Here's how the part is built. I have some questions about the finished solid (model axes, mm). Face numbers are marked on the shaded views. A direction names the side the tool comes from. Round coordinates to 2 decimals unless told otherwise and drop trailing zeros. Order: outer loops, then holes, each group sorted by start corner. A loop starts at its lowest first (then second) coordinate and runs counter-clockwise, first axis right, second up. Notation, with made-up numbers: (77, 22) -> (121, 22) arc R27 ccw to (121, 41) -> close; hole circle Ø1 at (71.25, -18). An arc over 180 degrees is marked (long way). Answer in a Markdown table with one row per item.
Solid Edge part; units mm, degrees
sketch "Sketch1" plane through (0, 0, 0) normal (0, 0, 1) x (1, 0, 0)
  line L0 (-22.86, 0) -> (22.86, 0)
  line L1 (22.86, 0) -> (22.86, 21.336)
  line L2 (22.86, 21.336) -> (-22.86, 21.336)
  line L3 (-22.86, 21.336) -> (-22.86, 0)
extrude "Protrusion1" add sketch "Sketch1" along normal blind 3.81
sketch "Sketch2" plane through (0, 10.668, 3.81) normal (0, 0, 1) x (1, 0, 0)
  circle A0 centre (12.7, 0) radius 8.001
  circle A1 centre (-12.7, 0) radius 8.001
  dimension "D1" = 12.7
  dimension "D2" = 12.7
extrude "ExtrudedProtrusion_2" add sketch "Sketch2" along normal blind 11.938
hole "Hole_1" at (20.32, 18.796, 3.81) direction (0, 0, -1) diameter 3.175 end up to next
hole "Hole1" at (-20.32, 2.54, 3.81) direction (0, 0, -1) diameter 3.175 end up to next
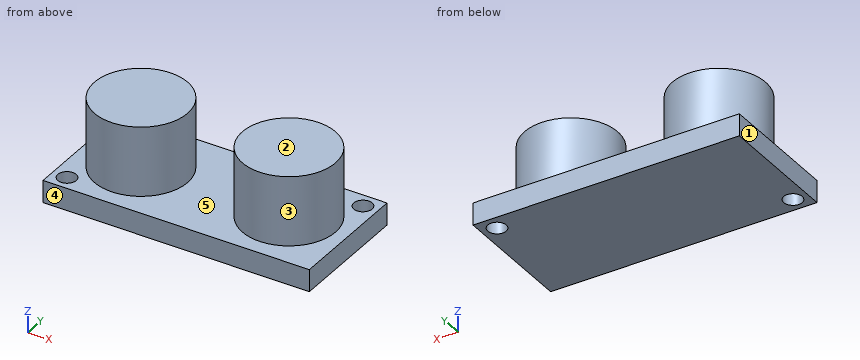
1. Suppose I cut it at A-A on y = 15.5. Write out the boundary of the cut face in (x, z), then the cut area to 3 significant figures.
Numbers:
| item | result |
|---|---|
| outline | (-22.86, 0) -> (22.86, 0) -> (22.86, 3.81) -> (19.08, 3.81) -> (19.08, 15.75) -> (6.32, 15.75) -> (6.32, 3.81) -> (-6.32, 3.81) -> (-6.32, 15.75) -> (-19.08, 15.75) -> (-19.08, 3.81) -> (-22.86, 3.81) -> close |
| area | 479 mm2 |
2. Suppose I cut it at C-C on z = 7. Write out the boundary of the cut face in (x, y).
Numbers:
| item | result |
|---|---|
| outline | circle Ø16 at (-12.7, 10.67); circle Ø16 at (12.7, 10.67) |
3. Suppose I cut it at D-D on x = 10. Write out the boundary of the cut face in (y, z), then the cut area to 3 significant figures.
Numbers:
| item | result |
|---|---|
| outline | (0, 0) -> (21.34, 0) -> (21.34, 3.81) -> (18.2, 3.81) -> (18.2, 15.75) -> (3.14, 15.75) -> (3.14, 3.81) -> (0, 3.81) -> close |
| area | 261 mm2 |
4. Please list where these lines run through material, in increasing order: line 1 along Y through (x, z) = (-20.32, 2.2); line 2 along Y through (x, z) = (20.32, 2.45); line 3 along X through (y, z) = (2.54, 1.2).
Numbers:
| item | result |
|---|---|
| line 1 | y = 0 to 0.95, 4.13 to 21.34 |
| line 2 | y = 0 to 17.21, 20.38 to 21.34 |
| line 3 | x = -22.86 to -21.91, -18.73 to 22.86 |
5. We'd pull the mould along X, two halves only. Please class the marked faces 1, 2 and 3: released by +X, released by -X, zero draft, split by the parting line, or undercut.
Numbers:
| item | result |
|---|---|
| face 1 | released by -X |
| face 2 | zero draft |
| face 3 | undercut |
6. For the marked faces 4 and 5, which set-ups out of +Z, -Z, +X, -X, +Y, -Y let a thin tool reach every point of the face, with its end or its side?
Numbers:
| item | result |
|---|---|
| face 4 | +Z, -Z, +X, -X, -Y |
| face 5 | +Z |
7. For pin 1 Ø1.5 at (y, z) = (16, 5) entering from -X; pin 2 Ø5 at (y, z) = (17.5, 8.5) entering from +X; pin 3 Ø4 at (x, z) = (8, 11.5) entering from -Y, each with a flat end and sliding along its axis, tell me the tip position at first contact or that it passes through.
Numbers:
| item | result |
|---|---|
| pin 1 | stops at x = -19.26 |
| pin 2 | stops at x = 19.43 |
| pin 3 | stops at y = 3.14 |
8. Suppose I cut it at B-B on x = -12.7. Write out the boundary of the cut face in (y, z).
Numbers:
| item | result |
|---|---|
| outline | (0, 0) -> (21.34, 0) -> (21.34, 3.81) -> (18.67, 3.81) -> (18.67, 15.75) -> (2.67, 15.75) -> (2.67, 3.81) -> (0, 3.81) -> close |
